```python
from build123d import *

# Parameters (mm, degrees)
SKETCH1_R           = 4
SKETCH1_R_2         = 1.85
BOSS_EXTRUDE1_DEPTH = 2


with BuildPart() as part:
    # Sketch1 → Boss-Extrude1 (new body)
    with BuildSketch(Plane(origin=(0, 0, 0), x_dir=(1, 0, 0), z_dir=(0, 1, 0))):
        with BuildLine():
            Line((-16, 13.5), (16, 13.5))
            ThreePointArc((16, 13.5), (29.5, 0), (16, -13.5))
            Line((16, -13.5), (-16, -13.5))
            ThreePointArc((-16, -13.5), (-29.5, 0), (-16, 13.5))
        make_face()
        Circle(SKETCH1_R, mode=Mode.SUBTRACT)
        with Locations((16, 0)):
            Circle(SKETCH1_R, mode=Mode.SUBTRACT)
        with Locations((8, 0)):
            Circle(SKETCH1_R_2, mode=Mode.SUBTRACT)
        with Locations((10.343145751, 5.656854249)):
            Circle(SKETCH1_R_2, mode=Mode.SUBTRACT)
        with Locations((16, 8)):
            Circle(SKETCH1_R_2, mode=Mode.SUBTRACT)
        with Locations((21.656854249, 5.656854249)):
            Circle(SKETCH1_R_2, mode=Mode.SUBTRACT)
        with Locations((24, 0)):
            Circle(SKETCH1_R_2, mode=Mode.SUBTRACT)
        with Locations((21.656854249, -5.656854249)):
            Circle(SKETCH1_R_2, mode=Mode.SUBTRACT)
        with Locations((16, -8)):
            Circle(SKETCH1_R_2, mode=Mode.SUBTRACT)
        with Locations((10.343145751, -5.656854249)):
            Circle(SKETCH1_R_2, mode=Mode.SUBTRACT)
        with Locations((-10.343145751, -5.656854249)):
            Circle(SKETCH1_R_2, mode=Mode.SUBTRACT)
        with Locations((-16, -8)):
            Circle(SKETCH1_R_2, mode=Mode.SUBTRACT)
        with Locations((-21.656854249, -5.656854249)):
            Circle(SKETCH1_R_2, mode=Mode.SUBTRACT)
        with Locations((-24, 0)):
            Circle(SKETCH1_R_2, mode=Mode.SUBTRACT)
        with Locations((-21.656854249, 5.656854249)):
            Circle(SKETCH1_R_2, mode=Mode.SUBTRACT)
        with Locations((-16, 8)):
            Circle(SKETCH1_R_2, mode=Mode.SUBTRACT)
        with Locations((-10.343145751, 5.656854249)):
            Circle(SKETCH1_R_2, mode=Mode.SUBTRACT)
        with Locations((-8, 0)):
            Circle(SKETCH1_R_2, mode=Mode.SUBTRACT)
        with Locations((-16, 0)):
            Circle(SKETCH1_R, mode=Mode.SUBTRACT)
    extrude(amount=BOSS_EXTRUDE1_DEPTH)


solid = part.part
```
Source: CAD feature listing. Evaluate the final solid. Frame: model axes, mm. Give positions to 0.01 mm unless a question says otherwise; leave off trailing zeros. Write each loop counter-clockwise with the first axis right and the second up, starting at its lowest first coordinate (ties: lowest second). Pieces come first, ordered by that corner, then holes.
1. First-contact query: pin 1 (4.5 mm diameter, centred on x = -21.66, z = -5.66, fed in from +Y); pin 2 (3 mm diameter, centred on x = 16, z = -8, fed in from +Y). Flat tips, straight axial feed; report the tip coordinate or a pass-through.
2. Section query C-C (z = 3). Return the cut outline in (x, y), then the cut area to 3 significant figures.
3. Pull-direction query (Z, two-part tool) for faces 1 (the face through (-29.497, 0.986, 0.297)), 2 (the face through (-23.505, 0.986, 5.576)), 3 (the face through (0, 1, -13.5)); classes: +Z half, -Z half, draft (parallel to the pull), parting line (faces both ways), or undercut.
4. Section query B-B (x = -21). Return the cut outline in (y, z).
5. Section query A-A (x = 19). Return the cut outline in (y, z), then the cut area to 3 significant figures.
6. Section query D-D (y = 1.2). Count the separate pieces of the cut face and the enclosed holes in it, then the cut area to 3 significant figures.
7. Material intervals for line 1 along Z through (x, y) = (10.5, 1.05); line 2 along Z through (x, y) = (-16, 0.5); line 3 along X through (y, z) = (1.3, 2), sorted ascending.
Output values:
1. pin 1: stops at y = 2
1. pin 2: passes through
2. outline: (-29.16, 0) - (-18.65, 0) - (-18.65, 2) - (-29.16, 2) - close; (-13.35, 0) - (-2.65, 0) - (-2.65, 2) - (-13.35, 2) - close; (2.65, 0) - (13.35, 0) - (13.35, 2) - (2.65, 2) - close; (18.65, 0) - (29.16, 0) - (29.16, 2) - (18.65, 2) - close
2. area: 84.9 mm2
3. face 1: parting line
3. face 2: undercut
3. face 3: -Z half
4. outline: (0, -12.54) - (2, -12.54) - (2, -7.39) - (0, -7.39) - close; (0, -3.93) - (2, -3.93) - (2, 3.93) - (0, 3.93) - close; (0, 7.39) - (2, 7.39) - (2, 12.54) - (0, 12.54) - close
5. outline: (0, -13.16) - (2, -13.16) - (2, -2.65) - (0, -2.65) - close; (0, 2.65) - (2, 2.65) - (2, 13.16) - (0, 13.16) - close
5. area: 42.1 mm2
6. separate pieces: 1
6. enclosed holes: 19
6. area: 1,110 mm2
7. line 1: z = -13.5 to -7.5, -3.81 to 3.81, 7.5 to 13.5
7. line 2: z = -13.5 to -9.85, -6.15 to -4, 4 to 6.15, 9.85 to 13.5
7. line 3: x = -29.35 to -19.46, -12.54 to -3.46, 3.46 to 12.54, 19.46 to 29.35
